from build123d import *

# Parameters (mm, degrees)
F0_W     = 44.45
F0_H     = 25.4
F1_DEPTH = 25.4
F2_W     = 31.75
F2_H     = 12.7
F3_DEPTH = 25.4
F5_DEPTH = 25.4
F6_W     = 12.7
F6_H     = 12.7
F7_DEPTH = 6.35
F8_R     = 6.35
F9_DEPTH = 12.7


with BuildPart() as f1:
    # F0 (on Front) → F1 (new body)
    with BuildSketch(Plane.XZ):
        with Locations((22.225, 12.7)):
            Rectangle(F0_W, F0_H)
    extrude(amount=F1_DEPTH)

    # F2 (on face) → F3 (cut)
    with BuildSketch(Plane.XY.offset(25.4)):
        with Locations((28.575, -19.05)):
            Rectangle(F2_W, F2_H)
    extrude(amount=-F3_DEPTH, mode=Mode.SUBTRACT)

    # F4 (on face) → F5 (cut)
    with BuildSketch(Plane.XZ.offset(12.7)):
        with BuildLine():
            ThreePointArc((28.575, 25.4), (41.275, 12.7), (28.575, 0))
            Line((28.575, 0), (44.45, 0))
            Line((44.45, 0), (44.45, 25.4))
            Line((44.45, 25.4), (28.575, 25.4))
        make_face()
    extrude(amount=-F5_DEPTH, mode=Mode.SUBTRACT)

    # F6 (on face) → F7 (cut)
    with BuildSketch(Plane.XZ.offset(25.4)):
        with Locations((6.35, 12.7)):
            Rectangle(F6_W, F6_H)
    extrude(amount=-F7_DEPTH, mode=Mode.SUBTRACT)

    # F8 (on face) → F9 (cut, through all)
    with BuildSketch(Plane.XZ.offset(12.7)):
        with Locations((25.4, 12.7)):
            Circle(F8_R)
    extrude(amount=-F9_DEPTH, mode=Mode.SUBTRACT)


solid = f1.part
Here's how the part is built. I have some questions about the finished solid (model axes, mm). A direction names the side the tool comes from. Round coordinates to 2 decimals unless told otherwise and drop trailing zeros. Loops run counter-clockwise (first coordinate to the right, second up) from the corner with the lowest first, then second, coordinate; pieces in that order, holes last. Notation, with made-up numbers: (-10, -35) -> (-1, -35) arc R24 cw to (-1, -3) -> close; hole circle Ø4 at (-12.75, 5.5). An arc over 180 degrees is marked (long way). Write each question's results on one line, items separated by ' | '.
(1) For P1, Ø12.5, axis at x = 23, z = 7.5, coming from the -Y side; P2, Ø6.5, axis at y = -19, z = 15.5, coming from the +X side; P3, Ø4, axis at x = 14.5, z = 13, coming from the -Y side; P4, Ø1, axis at y = -20, z = 10, coming from the -X side, each with a flat end and sliding along its axis, tell me the tip position at first contact or that it passes through.
Worked answers:
P1: y = -12.7 | P2: x = 12.7 | P3: y = -19.05 | P4: through
(2) If I drill on L1, parallel to Z at x = 25.4, y = -5.75; L2, parallel to Y at x = 28.5, z = 21.5; L3, parallel to X at y = -20.5, z = 2.5, over which ranges is the centre line in solid material (lowest first)?
Worked answers:
L1: 0 to 6.35, 19.05 to 25.4 | L2: -12.7 to 0 | L3: 0 to 12.7
(3) If we section it at B-B, the plane x = 25.4: List the corners of the cut face in (y, z) for me.
Worked answers:
outline: (-12.7, 0) -> (0, 0) -> (0, 6.35) -> (-12.7, 6.35) -> close; (-12.7, 19.05) -> (0, 19.05) -> (0, 25.4) -> (-12.7, 25.4) -> close
(4) If we section it at A-A, the plane z = 12.7: List the corners of the cut face in (x, y) for me (3 decimals).
Worked answers:
outline: (0, -19.05) -> (12.7, -19.05) -> (12.7, -12.7) -> (19.05, -12.7) -> (19.05, 0) -> (0, 0) -> close; (31.75, -12.7) -> (41.275, -12.7) -> (41.275, 0) -> (31.75, 0) -> close
(5) If we section it at D-D, the plane z = 8: List the corners of the cut face in (x, y) for me, then the cut area to 3 significant figures.
Worked answers:
outline: (0, -19.05) -> (12.7, -19.05) -> (12.7, -12.7) -> (21.13, -12.7) -> (21.13, 0) -> (0, 0) -> close; (29.67, -12.7) -> (40.37, -12.7) -> (40.37, 0) -> (29.67, 0) -> close | area: 485 mm2
(6) If we section it at C-C, the plane x = 11: List the corners of the cut face in (y, z) for me.
Worked answers:
outline: (-25.4, 0) -> (0, 0) -> (0, 25.4) -> (-25.4, 25.4) -> (-25.4, 19.05) -> (-19.05, 19.05) -> (-19.05, 6.35) -> (-25.4, 6.35) -> close
(7) For faces 5 (the face through (12.7, -18, 13)), 6 (the face through (6, -22, 6.35)), 7 (the face through (20.72, -6.44, 16.99)), which set-ups out of +Z, -Z, +X, -X, +Y, -Y let a thin tool reach every point of the face, with its end or its side?
Worked answers:
face 5: +Z, -Z, +X, -Y | face 6: +X, -X, -Y | face 7: +Y, -Y
(8) We'd pull the mould along Z, two halves only. Please class faces 1 (the face through (6, -25.4, 22)), 2 (the face through (6, -19.05, 13)), 3 (the face through (41.27, -6.44, 12.98)), 4 (the face through (6, -22, 19.05)): released by +Z, released by -Z, zero draft, split by the parting line, or undercut.
Worked answers:
face 1: zero draft | face 2: undercut | face 3: split by the parting line | face 4: undercut
